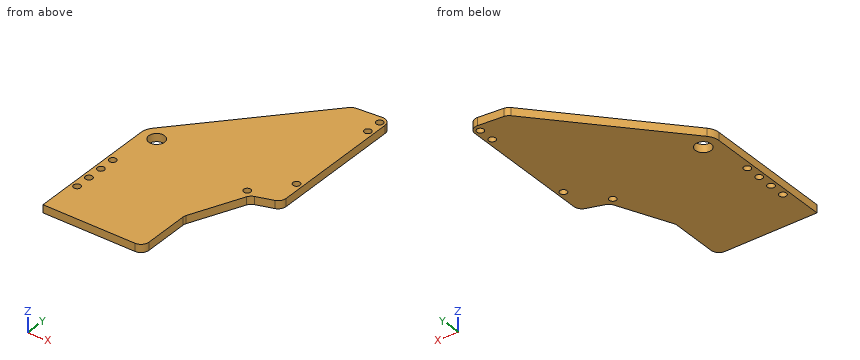
Autodesk Inventor part; units mm, degrees
ref_plane "YZ Plane" through (0, 0, 0) normal (1, 0, 0) x (0, 1, 0)
ref_plane "XZ Plane" through (0, 0, 0) normal (0, 1, 0) x (-1, 0, 0)
ref_plane "XY Plane" through (0, 0, 0) normal (0, 0, 1) x (1, 0, 0)
sketch "Sketch1" plane through (0, 0, 0) normal (0, 0, 1) x (1, 0, 0)
  line L0 (0, 0) -> (0, 136.525)
  line L1 (-11.7886, 12.2907) -> (-39.6863, 18.4755) construction
  line L2 (-39.6863, 18.4755) -> (-33.3297, 47.1481) construction
  line L3 (-33.3297, 47.1481) -> (-5.432, 40.9633) construction
  line L4 (-5.432, 40.9633) -> (-11.7886, 12.2907) construction
  line L5 (-39.6863, 18.4755) -> (-5.432, 40.9633) construction
  line L6 (-33.3297, 47.1481) -> (-11.7886, 12.2907) construction
  circle A0 centre (-53.975, 12.7) radius 3.175
  circle A1 centre (-53.975, 12.7) radius 6.35
  line L7 (0, 0) -> (-54.712, 6.3929) construction
  line L8 (-59.6703, 15.5082) -> (0, 136.525) construction
  line L9 (-27.1302, 45.7737) -> (-37.4529, 28.5497) construction
  line L10 (-11.6315, 42.3377) -> (-9.5552, 22.3649) construction
  line L11 (-19.3809, 44.0557) -> (-25.7374, 15.3831) construction
  line L12 (0, 92.075) -> (-19.7574, 96.4551) construction
  line L13 (-35.3766, 8.5768) -> (-19.8779, 5.1408) construction
  line L14 (-19.8779, 5.1408) -> (-21.2523, -1.0586) construction
  line L15 (-21.2523, -1.0586) -> (-36.751, 2.3773) construction
  line L16 (-36.751, 2.3773) -> (-35.3766, 8.5768) construction
  line L17 (-35.3766, 8.5768) -> (-41.27, 4.8223) construction
  line L18 (-19.8779, 5.1408) -> (-17.9381, 2.096) construction
  line L19 (-5.432, 40.9633) -> (-33.3297, 47.1481) construction
  line L20 (-33.3297, 47.1481) -> (-32.2475, 52.0296) construction
  line L21 (-32.2475, 52.0296) -> (-4.3498, 45.8448) construction
  line L22 (-4.3498, 45.8448) -> (-5.432, 40.9633) construction
  line L23 (-53.2878, 15.7997) -> (-53.975, 12.7) construction
  line L24 (-53.975, 12.7) -> (-57.0747, 13.3872) construction
  line L25 (-27.6272, 6.8588) -> (-34.4992, -24.1386) construction
  line L26 (-31.8676, 50.076) -> (-5.5198, 44.2349) construction
  line L27 (-5.5198, 44.2349) -> (-4.489, 48.8845) construction
  line L28 (-4.489, 48.8845) -> (-30.8368, 54.7256) construction
  line L29 (-30.8368, 54.7256) -> (-31.8676, 50.076) construction
  line L30 (-31.3522, 52.4008) -> (-5.0044, 46.5597) construction
  circle A2 centre (-29.0274, 51.8854) radius 1.4732 construction
  circle A3 centre (-22.8279, 50.5111) radius 1.4732 construction
  circle A4 centre (-16.6284, 49.1367) radius 1.4732 construction
  circle A5 centre (-10.4289, 47.7623) radius 1.4732 construction
  circle A6 centre (-10.3614, 84.7398) radius 1.4732 construction
  line L31 (-53.975, 12.7) -> (-13.3751, 95.0402) construction
  line L32 (-32.2923, 56.6744) -> (0, 49.5153) construction
  circle A7 centre (-10.3614, 84.7398) radius 4.7625 construction
  line L33 (-4.7625, 50.5712) -> (-4.7625, 93.1308) construction
  line L34 (-27.5056, 55.6132) -> (-14.3936, 82.2055) construction
  line L35 (-5.6003, 84.6261) -> (-4.7625, 84.4403) construction
  line L36 (-17.9381, 2.096) -> (0, 2.096) construction
  line L37 (0, 2.096) -> (0, -1.079) construction
  line L38 (0, -1.079) -> (-17.9381, -1.079) construction
  line L39 (-17.9381, -1.079) -> (-17.9381, 2.096) construction
  circle A8 centre (-12.7, 7.9375) radius 1.5875 construction
  line L40 (-12.7, 7.9375) -> (0, 7.9375) construction
  line L41 (0, 7.9375) -> (-17.9381, 2.096)
  circle A9 centre (-12.7, 7.9375) radius 3.175 construction
  line L42 (-9.525, 7.9375) -> (-9.525, 4.8357) construction
  line L43 (-9.525, 7.9375) -> (0, 7.9375) construction
  line L44 (-17.9187, 46.9837) -> (-16.8879, 51.6333) construction
  line L45 (-12.4942, 45.7811) -> (-26.2381, -16.2137) construction
  line L46 (0, 66.675) -> (0, 7.9375) construction
  line L47 (-26.2381, -16.2137) -> (-20.0386, -17.5881) construction
  line L48 (-20.0386, -17.5881) -> (-8.7313, 7.9375)
  circle A10 centre (-12.7, 6.35) radius 1.4224
  line L49 (0, 13.4938) -> (-4.7625, 13.4938) construction
  line L50 (-4.7625, 13.4938) -> (-4.7625, 24.6063) construction
  line L51 (-4.7625, 24.6063) -> (0, 24.6063) construction
  line L52 (0, 24.6063) -> (0, 13.4938) construction
  line L53 (-4.7625, 19.05) -> (0, 19.05) construction
  circle A11 centre (-2.3813, 19.05) radius 1.4224
  line L54 (-20.7405, 8.5842) -> (-9.7454, 58.18) construction
  line L55 (-9.7454, 58.18) -> (-3.5459, 56.8056) construction
  line L56 (-3.5459, 56.8056) -> (-14.5411, 7.2098) construction
  line L57 (-14.5411, 7.2098) -> (-20.7405, 8.5842) construction
  line L58 (-12.7, 6.35) -> (-12.7, 7.9375) construction
  line L59 (-11.5442, 1.5875) -> (-9.525, 1.5875) construction
  line L60 (-9.525, 1.5875) -> (-9.525, 7.9375) construction
  line L61 (-9.525, 7.9375) -> (-11.5442, 7.9375) construction
  line L62 (-11.5442, 7.9375) -> (-11.5442, 1.5875) construction
  line L63 (-9.7454, 58.18) -> (-15.9449, 59.5544) construction
  line L64 (-15.9449, 59.5544) -> (-14.6504, 65.3933) construction
  line L65 (-14.6504, 65.3933) -> (0, 66.675)
  line L66 (-9.7454, 58.18) -> (-17.3193, 53.3549) construction
  arc A12 (-10.2313, 55.9882) -> (-11.9373, 58.6659) centre (-11.0843, 57.3271) ccw construction
  line L67 (-4.7625, 57.15) -> (0, 57.15) construction
  circle A13 centre (-2.3813, 57.15) radius 1.4224
  circle A14 centre (-2.3813, 63.5) radius 1.4224
  line L68 (0, 7.9375) -> (-60.325, 7.9375) construction
  line L69 (-60.325, 7.9375) -> (-60.325, -39.6875) construction
  line L70 (-60.325, -39.6875) -> (0, -39.6875)
  line L71 (0, -39.6875) -> (0, 7.9375)
  line L72 (-60.325, -39.6875) -> (-60.325, 12.7)
  line L73 (-58.6735, 16.9717) -> (-14.6504, 65.3933)
  line L74 (-60.325, -30.1625) -> (-60.325, -3.175) construction
  line L75 (-60.325, -3.175) -> (-55.5625, -3.175) construction
  line L76 (-55.5625, -3.175) -> (-55.5625, -30.1625) construction
  line L77 (-55.5625, -30.1625) -> (-60.325, -30.1625) construction
  line L78 (-60.325, -24.6062) -> (-55.5625, -24.6062) construction
  circle A15 centre (-57.9437, -24.6063) radius 1.4224
  circle A16 centre (-57.9437, -18.2563) radius 1.4224
  circle A17 centre (-57.9437, -11.9063) radius 1.4224
  circle A18 centre (-57.9437, -5.5563) radius 1.4224
  line L79 (-20.0386, -17.5881) -> (-20.0386, -39.6875)
  point P0 (-22.5591, 29.7194)
  point P1 (-20.4869, 2.3938)
  point P2 (-36.3367, 4.2458)
  point P3 (-51.1668, 18.3953)
  point P4 (-11.1125, 7.9375)
  point P5 (-11.4283, 6.9872)
  point P6 (-11.9574, 7.9375)
  point P7 (-13.9717, 6.9872)
  point P8 (-9.525, 6.1457)
  point P9 (-10.2031, 4.6149)
  dimension "d74" = 6.35
  dimension "d13" = 136.525
  dimension "d14" = 29.3687
  dimension "d15" = 28.575
  dimension "d16" = 12.5
  dimension "d17" = 6.35
  dimension "d19" = 53.975
  dimension "d22" = 12.7
  dimension "d23" = 7.9375
  dimension "d24" = 19.05
  dimension "d26" = 102.5
  dimension "d29" = 6.35
  dimension "d31" = 7.9375
  dimension "d34" = 5
  dimension "d35" = 26.9875
  dimension "d38" = 31.75
  dimension "d40" = 26.9875
  dimension "d41" = 4.7625
  dimension "d42" = 2.9464
  dimension "d43" = 2.3813
  dimension "d46" = 6.35
  dimension "d51" = 2.9464
  dimension "d52" = 79.7719
  dimension "d53" = 6.35
  dimension "d54" = 9.525
  dimension "d55" = 4.7625
  dimension "d56" = 4.7625
  dimension "d60" = 12.7
  dimension "d61" = 3.175
  dimension "d63" = 3.175
  dimension "d66" = 3.175
  dimension "d67" = 12.7
  dimension "d72" = 8.7312
  dimension "d73" = 7.9375
  dimension "d75" = 34.925
  dimension "d80" = 12.7
  dimension "d82" = 7.9375
  dimension "d83" = 63.5
  dimension "d84" = 66.675
  dimension "d85" = 6.35
  dimension "d86" = 92.075
  dimension "d87" = 2.8448
  dimension "d88" = 4.7625
  dimension "d89" = 11.1125
  dimension "d90" = 2.8448
  dimension "d91" = 19.05
  dimension "d92" = 6.35
  dimension "d93" = 50.8
  dimension "d94" = 25.4
  dimension "d95" = 8.7312
  dimension "d96" = 9.525
  dimension "d97" = 6.35
  dimension "d99" = 6.35
  dimension "d101" = 3.175
  dimension "d106" = 2.8448
  dimension "d107" = 57.15
  dimension "d110" = 6.35
  dimension "d119" = 85
  dimension "d121" = 47.625
  dimension "d123" = 4.7625
  dimension "d124" = 26.9875
  dimension "d125" = 9.525
  dimension "d126" = 2.8448
  dimension "d130" = 6.35
  dimension "d135" = 2.3813
extrude "Extrusion1" add sketch "Sketch1" along normal blind 3.175 contours L41 L48 L79 L70 L72 A1 L73 L65 L0 | A1
fillet "Fillet5" radius 3.175 6 edges at (-14.6504, 65.3933, 1.5875) (0, 66.675, 1.5875) (-20.0386, -39.6875, 1.5875) (-20.0386, -17.5881, 1.5875) (-10.2031, 4.6149, 1.5875) (0, 7.9375, 1.5875)
equation "\"d56\" = d55"
properties part number "Uprights" material "UHMW, White"
Source: CAD feature listing. Evaluate the final solid. Frame: model axes, mm. Give positions to 0.01 mm unless a question says otherwise; leave off trailing zeros. Loops run counter-clockwise (first coordinate to the right, second up) from the corner with the lowest first, then second, coordinate; pieces in that order, holes last. Notation, with made-up numbers: M 78,16 L 117,16 A5 ccw 117,21 Z; hole C 50,31.5 d1. An arc over 180 degrees is marked long. Put each result on its own line as item: value.
Q1. Section C-C (y = 19.05). Return the cut outline in (x, z) (3 decimals), and give its area (3 significant figures).
Response values:
outline: M -56.784,0 L -3.804,0 L -3.804,3.175 L -56.784,3.175 Z; M -0.959,0 L 0,0 L 0,3.175 L -0.959,3.175 Z
area: 171 mm²
Q2. Section D-D (x = -47). Return the cut outline in (y, z) (1 decimal).
Response values:
outline: M -39.7,0 L 29.8,0 L 29.8,3.2 L -39.7,3.2 Z
Q3. Line query: probe 1 along Y at (x, z) = (-56, 2.4); probe 2 along Y at (x, z) = (-12.7, 1.35); probe 3 along X at (y, z) = (-30, 0.8) (3 decimals). Output: solid intervals per line, ascending. Write a range as [from, to].
Response values:
probe 1: y = [-39.69, 10.25], [15.15, 19.91]
probe 2: y = [-1.02, 4.93], [7.77, 65.56]
probe 3: x = [-60.325, -20.039]
Q4. Section B-B (z = 1.9). Count the separate pieces of the cut face and the enclosed holes in it, and give its area (3 significant figures).
Response values:
separate pieces: 1
enclosed holes: 9
area: 4,320 mm²
Q5. Pin query (flat end, axial travel): P1, Ø3.5, axis at x = -57.94, y = -24.61, coming from the -Z side; P2, Ø2.5, axis at x = -12.7, y = 6.35, coming from the +Z side. Return the tip coordinate at first contact, or that it passes through.
Response values:
P1: stops at z = 0
P2: passes through
Q6. Section A-A (y = 57.15). Return the cut outline in (x, z) (3 decimals).
Response values:
outline: M -22.145,0 L -3.804,0 L -3.804,3.175 L -22.145,3.175 Z; M -0.959,0 L 0,0 L 0,3.175 L -0.959,3.175 Z
